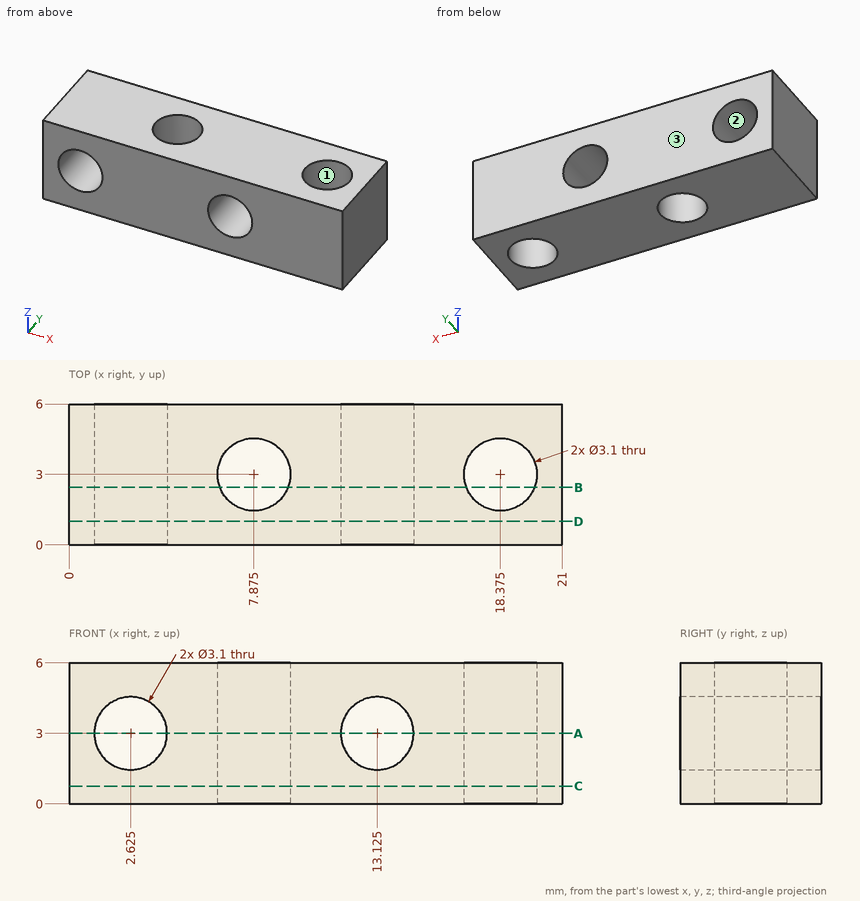
Source: three-view drawing plus pictorial views. Frame: mm from the lowest corner of the part. Give positions to 0.01 mm unless a question says otherwise; leave off trailing zeros. Order: outer loops, then holes, each group sorted by start corner. A loop starts at its lowest first (then second) coordinate and runs counter-clockwise, first axis right, second up. Notation, with made-up numbers: (13.25, -26.5) - (60.25, -26.5) arc R18 cw to (60.25, -18.5) - close; hole circle Ø1 at (44.25, -2.75). An arc over 180 degrees is marked (long way). Answer as a JSON object with one key per item and string values. Group by question number.
Q1. Cut plane B-B, the plane y = 2.45. Output: boundary loops of the cut face in (x, z) (3 decimals).
Q2. Cut plane C-C, the plane z = 0.75. Output: boundary loops of the cut face in (x, y) (3 decimals).
Q3. Cut plane A-A, the plane z = 3. Output: boundary loops of the cut face in (x, y) (3 decimals), then the cut area to 3 significant figures.
Q4. Line query: probe 1 along Z at (x, y) = (2.75, 0.8); probe 2 along X at (y, z) = (3.1, 2.3). Output: solid intervals per line, ascending.
Q5. Mould query, pull axis Y, two halves, no side actions, for the marked faces 1, 2 and 3. Classes: pulls with the +Y half, pulls with the -Y half, needs draft (parallel to the pull), parting line crosses it, or undercut.
Q6. Cut plane D-D, the plane y = 1. Output: boundary loops of the cut face in (x, z) (3 decimals), then the cut area to 3 significant figures.
Results:
{
 "1": {"outline": "(0, 0) - (6.426, 0) - (6.426, 6) - (0, 6) - close; (9.324, 0) - (16.926, 0) - (16.926, 6) - (9.324, 6) - close; (19.824, 0) - (21, 0) - (21, 6) - (19.824, 6) - close; hole circle Ø3.1 at (2.625, 3); hole circle Ø3.1 at (13.125, 3)"},
 "2": {"outline": "(0, 0) - (21, 0) - (21, 6) - (0, 6) - close; hole circle Ø3.1 at (7.875, 3); hole circle Ø3.1 at (18.375, 3)"},
 "3": {"outline": "(0, 0) - (1.075, 0) - (1.075, 6) - (0, 6) - close; (4.175, 0) - (11.575, 0) - (11.575, 6) - (4.175, 6) - close; (14.675, 0) - (21, 0) - (21, 6) - (14.675, 6) - close; hole circle Ø3.1 at (7.875, 3); hole circle Ø3.1 at (18.375, 3)", "area": "73.7 mm^2"},
 "4": {"probe 1": "0 to 1.46, 4.54 to 6", "probe 2": "0 to 1.24, 4.01 to 6.33, 9.42 to 11.74, 14.51 to 16.83, 19.92 to 21"},
 "5": {"face 1": "undercut", "face 2": "needs draft", "face 3": "pulls with the +Y half"},
 "6": {"outline": "(0, 0) - (21, 0) - (21, 6) - (0, 6) - close; hole circle Ø3.1 at (2.625, 3); hole circle Ø3.1 at (13.125, 3)", "area": "111 mm^2"}
}
